Geometry: final body of the model. Coordinates: model frame, mm. A direction names the side the tool comes from. Give positions to 0.01 mm unless a question says otherwise; leave off trailing zeros. Loops run counter-clockwise (first coordinate to the right, second up) from the corner with the lowest first, then second, coordinate; pieces in that order, holes last. Notation, with made-up numbers: (73, 28.25) - (100, 28.25) arc R16 cw to (100, 54.25) - close; hole circle Ø2 at (54.25, -11). An arc over 180 degrees is marked (long way). Use one line per item in the form item = value.
```python
from build123d import *

# Parameters (mm, degrees)
F0_W      = 12.5012692667
F0_H      = 25
F1_DEPTH  = 2.5
F2_W      = 2.5
F2_H      = 20
F2_H_2    = 2.5
F2_H_3    = 27.5
F3_DEPTH  = 22
F4_DEPTH  = 5
F5_R      = 2.25
F6_DEPTH  = 25
F9_DEPTH  = 5
F11_DEPTH = 25


with BuildPart() as f1:
    # F0 (on Top) → F1 (new body)
    with BuildSketch(Plane.XY):
        with Locations((-3.4478325397, 12.5846065283)):
            Rectangle(F0_W, F0_H)
        with BuildLine():
            Line((-1.6978325397, 19.8346065283), (-1.6978325397, 11.8346065283))
            ThreePointArc((-1.6978325397, 11.8346065283), (-3.4478325397, 10.0846065283), (-5.1978325397, 11.8346065283))
            Line((-5.1978325397, 11.8346065283), (-5.1978325397, 19.8346065283))
            ThreePointArc((-5.1978325397, 19.8346065489), (-3.4478325254, 21.5846065283), (-1.6978325397, 19.8346065205))
        make_face(mode=Mode.SUBTRACT)
    extrude(amount=F1_DEPTH)

    # F2 (on face) → F3 (join)
    with BuildSketch(Plane.XZ.offset(-0.0846065283)):
        with Locations((1.5528020937, 12.5)):
            Rectangle(F2_W, F2_H)
        with Locations((1.5528020937, 1.25)):
            Rectangle(F2_W, F2_H_2)
        with Locations((1.5528020937, -13.75)):
            Rectangle(F2_W, F2_H_3)
    extrude(amount=F3_DEPTH)

    # F4 (add): a face of the model
    f4_faces = [f1.faces().sort_by_distance(p)[0] for p in [
        (1.5528020937, 0.0846065283, 12.5),
    ]]
    extrude(f4_faces, amount=F4_DEPTH)

    # F5 (on face) → F6 (cut)
    with BuildSketch(Plane(origin=(0.3028020937, 0, 0), x_dir=(0, -1, 0), z_dir=(-1, 0, 0))):
        with Locations((10.9153934717, 12.5)):
            Circle(F5_R)
    extrude(amount=-F6_DEPTH, mode=Mode.SUBTRACT)

    # F8 (on offset) → F9 (join)
    with BuildSketch(Plane.XZ.offset(-0.0846065283)):
        Polygon((0.3028020937, 12.5), (-9.698467173, 2.5), (0.3028020937, 2.5), align=None)
    extrude(amount=-F9_DEPTH)

    # F10 (on face) → F11 (cut)
    with BuildSketch(Plane(origin=(0, 5.0846065283, 0), x_dir=(-1, 0, 0), z_dir=(0, 1, 0))):
        with BuildLine():
            Line((9.698467173, 2.5), (-0.3028020937, 12.5))
            ThreePointArc((-0.3028020937, 12.5), (3.1881480162, 5.9901238573), (9.698467173, 2.5))
        make_face()
    extrude(amount=-F11_DEPTH, mode=Mode.SUBTRACT)


solid = f1.part
```
(1) Material intervals for L1, parallel to Y at x = 1.25, z = 17.5; L2, parallel to X at y = -17, z = -1.5; L3, parallel to Y at x = -7, z = 1.5, sorted ascending. Write a range as from..to.
Solution:
L1 = -21.92..5.08
L2 = 0.3..2.8
L3 = 0.08..25.08
(2) Pull-direction query (Y, two-part tool) for faces 1 (the face through (-3.486, 21.584, 1.232)), 2 (the face through (-9.698, 12, 1)), 3 (the face through (-4, 25.085, 1)); classes: released by +Y, released by -Y, zero draft, split by the parting line, or undercut.
Solution:
face_1 = undercut
face_2 = zero draft
face_3 = released by +Y
(3) Cut plane B-B (x = -7). Return the cut outline in (y, z), plus the area to 3 significant figures.
Solution:
outline = (0.08, 0) - (25.08, 0) - (25.08, 2.5) - (5.08, 2.5) - (5.08, 3.36) - (0.08, 3.36) - close
area = 66.8 mm2
(4) Access query for faces 4 (the face through (-4, 10, 0)), 5 (the face through (-4, 0.085, 4)), 6 (the face through (-1.698, 16, 1)), 7 (the face through (0, 5.085, 10)), 8 (the face through (2, -21.915, -2)). Directions: +Z, -Z, +X, -X, +Y, -Y. A direction counts if a zero-diameter tool reaches every point of the face in a straight line with its end or side. Return the directions, or none.
Solution:
face_4 = -Z, +X, -X, +Y
face_5 = +Z, -Z, -X, -Y
face_6 = +Z, -Z
face_7 = +Z, +X, -X, +Y
face_8 = +Z, -Z, +X, -X, -Y
(5) Cut plane D-D (y = -1). Return the cut outline in (x, z), plus the area to 3 significant figures.
Solution:
outline = (0.3, -27.5) - (2.8, -27.5) - (2.8, 22.5) - (0.3, 22.5) - close
area = 125 mm2
(6) Cut plane A-A (y = 21). Return the cut outline in (x, z), plus the area to 3 significant figures.
Solution:
outline = (-9.7, 0) - (-4.75, 0) - (-4.75, 2.5) - (-9.7, 2.5) - close; (-2.14, 0) - (2.8, 0) - (2.8, 2.5) - (-2.14, 2.5) - close
area = 24.7 mm2
(7) Pin query (flat end, axial travel): P1, Ø5, axis at x = -5.5, z = 8.5, coming from the -Y side; P2, Ø3, axis at x = 0.5, z = -15.5, coming from the +Y side; P3, Ø6.5, axis at x = -2.5, y = 18, coming from the -Z side; P4, Ø2, axis at x = -8, y = 20.5, coming from the +Z side. Return the tip coordinate at first contact, or that it passes through.
Solution:
P1 = through
P2 = 0.08
P3 = 0
P4 = 2.5
(8) Cut plane C-C (z = 8). Return the cut outline in (x, y).
Solution:
outline = (-1.55, 0.08) - (0.3, 0.08) - (0.3, -21.92) - (2.8, -21.92) - (2.8, 5.08) - (-1.55, 5.08) - close
